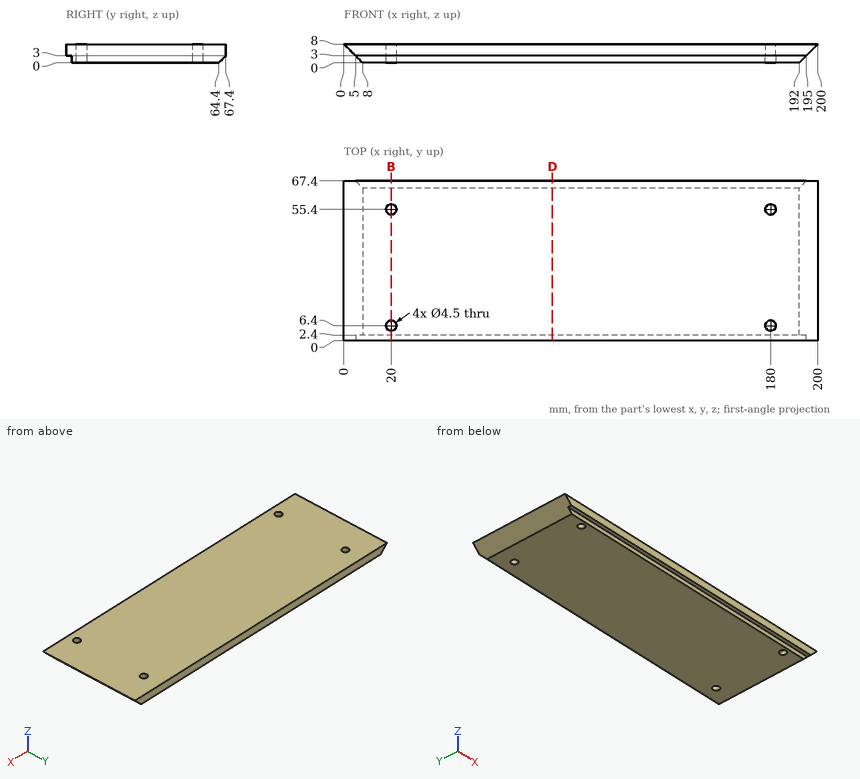
Answer from the drawing. Dimensions are ordinates in mm from the lowest x, y and z of the part. Coordinates: 2 decimals unless noted, no trailing zeros. Loops run counter-clockwise (first coordinate to the right, second up) from the corner with the lowest first, then second, coordinate; pieces in that order, holes last. Notation, with made-up numbers: (63.25, 46.25) - (103.25, 46.25) arc R15 ccw to (103.25, 60.25) - close; hole circle Ø8 at (-5.5, 33). An arc over 180 degrees is marked (long way). Use a Markdown table: item, result.
Item 1: Find section D-D, the plane x = 88. Determine the outline of the cut face in (y, z), and give its area (4 significant figures).
Evaluation:
| item | result |
|---|---|
| outline | (0, 3) - (2.4, 3) - (2.4, 0) - (64.4, 0) - (67.4, 3) - (67.4, 8) - (0, 8) - close |
| area | 527.5 mm2 |
Item 2: Find section B-B, the plane x = 20. Determine the outline of the cut face in (y, z).
Evaluation:
| item | result |
|---|---|
| outline | (0, 3) - (2.4, 3) - (2.4, 0) - (4.15, 0) - (4.15, 8) - (0, 8) - close; (8.65, 0) - (53.15, 0) - (53.15, 8) - (8.65, 8) - close; (57.65, 0) - (64.4, 0) - (67.4, 3) - (67.4, 8) - (57.65, 8) - close |
Item 3: Consider probe 1 along Y at (x, z) = (20, 5.65); probe 2 along Y at (x, z) = (20, 1.15); probe 3 along X at (y, z) = (7.5, 5). Determine where each line is inside the solid, lowest interval first. Write a range as from..to.
Evaluation:
| item | result |
|---|---|
| probe 1 | y = 0..4.15, 8.65..53.15, 57.65..67.4 |
| probe 2 | y = 2.4..4.15, 8.65..53.15, 57.65..65.55 |
| probe 3 | x = 3..18.04, 21.96..178.04, 181.96..197 |
Item 4: Given pin 1 Ø0.7 at (x, y) = (125.5, 1.5) entering from -Z; pin 2 Ø2.5 at (x, y) = (20, 55.4) entering from +Z; pin 3 Ø7 at (x, y) = (20, 6.4) entering from +Z; pin 4 Ø1.5 at (y, z) = (19, 4.5) entering from +X, each flat-ended and moving along its own axis, determine where each tip first touches the part or whether it passes through.
Evaluation:
| item | result |
|---|---|
| pin 1 | stops at z = 3 |
| pin 2 | passes through |
| pin 3 | stops at z = 8 |
| pin 4 | stops at x = 197.25 |
